The listing builds one solid part. Answer for the finished solid, in the listing's coordinates (mm). Face numbers are marked on the shaded views. A direction names the side the tool comes from. Round coordinates to 2 decimals unless told otherwise and drop trailing zeros. Order: outer loops, then holes, each group sorted by start corner. A loop starts at its lowest first (then second) coordinate and runs counter-clockwise, first axis right, second up. Notation, with made-up numbers: (78.5, -26.75) - (85.5, -26.75) arc R15 ccw to (85.5, -14.75) - close; hole circle Ø10 at (82, 85). An arc over 180 degrees is marked (long way). One line per item, written item: value. Start each with the question number.
1. Section D-D, the plane z = 9.5 is taken. Give the vertices of the cut face in (x, y), then the cut area to 3 significant figures.
2. A tool of negligible diameter and unlimited length cuts with its end or side. For the marked faces 5, 6, 7 and 8, from which of +Z, -Z, +X, -X, +Y, -Y can it reach the whole face along a straight path? Write none if from no direction.
3. Section C-C, the plane y = -0.3 is taken. Give the vertices of the cut face in (x, z).
4. Section B-B, the plane z = -13 is taken. Give the vertices of the cut face in (x, y), then the cut area to 3 significant figures.
5. For a pull along Z with two mould halves and no side action, classify the marked faces 1, 2, 3 and 4 as released by +Z, released by -Z, zero draft, split by the parting line, or undercut.
6. Section A-A, the plane x = 5 is taken. Give the vertices of the cut face in (y, z).
7. Flat-ended cylindrical pins translate along their axes: P1, Ø1.5, axis at y = -0.5, z = 3, coming from the -X side; P2, Ø1.5, axis at x = -7.5, y = 0, coming from the +Z side; P3, Ø1.5, axis at y = -0.5, z = 16, coming from the +X side; P4, Ø4, axis at x = 5, z = 9.5, coming from the +Y side. Find the tip coordinate at first contact, or state that the pin passes through.
8. Straight lines are drawn through the part: line 1 (X direction, y = -0.8, z = 9.5); line 2 (Z direction, x = 1.75, y = -0.95); line 3 (Z direction, x = 5, y = 0.55). For each, find the intervals that lie inside material, in ascending order.
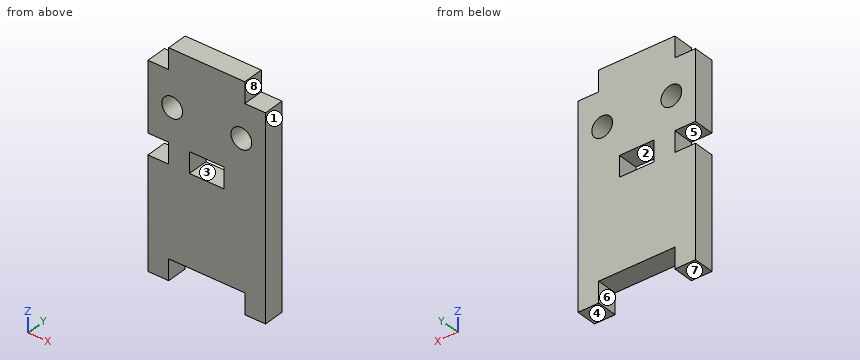
from build123d import *

# Parameters (mm, degrees)
SKETCH1_W               = 17
SKETCH1_H               = 29
BOSS_EXTRUDE1_DEPTH     = 1.5
SKETCH2_W               = 11
SKETCH2_H               = 3
BOSS_EXTRUDE2_DEPTH     = 1.5
SKETCH3_W               = 5
SKETCH3_H               = 3
SKETCH3_W_2             = 11
SKETCH3_W_3             = 3
CUT_EXTRUDE1_DEPTH      = 2.5
CUT_EXTRUDE1_DEPTH_BACK = 2.5
SKETCH5_R               = 1.5
CUT_EXTRUDE3_DEPTH      = 2.5
CUT_EXTRUDE3_DEPTH_BACK = 2.5


with BuildPart() as part:
    # Sketch1 → Boss-Extrude1 (new body, symmetric)
    with BuildSketch(Plane(origin=(0, 0, 0), x_dir=(1, 0, 0), z_dir=(0, 1, 0))):
        Rectangle(SKETCH1_W, SKETCH1_H)
    extrude(amount=BOSS_EXTRUDE1_DEPTH, both=True)

    # Sketch2 → Boss-Extrude2 (add, symmetric)
    with BuildSketch(Plane(origin=(0, 0, 0), x_dir=(1, 0, 0), z_dir=(0, 1, 0))):
        with Locations((0, -16)):
            Rectangle(SKETCH2_W, SKETCH2_H)
    extrude(amount=BOSS_EXTRUDE2_DEPTH, both=True)

    # Sketch3 → Cut-Extrude1 (cut, two sides)
    with BuildSketch(Plane(origin=(0, 0, 0), x_dir=(1, 0, 0), z_dir=(0, 1, 0))) as cut_extrude1_sk:
        with Locations((0, -3)):
            Rectangle(SKETCH3_W, SKETCH3_H)
        with Locations((0, 13)):
            Rectangle(SKETCH3_W_2, SKETCH3_H)
        with Locations((-7, -3)):
            Rectangle(SKETCH3_W_3, SKETCH3_H)
    extrude(amount=CUT_EXTRUDE1_DEPTH, mode=Mode.SUBTRACT)
    extrude(cut_extrude1_sk.sketch, amount=-CUT_EXTRUDE1_DEPTH_BACK, mode=Mode.SUBTRACT)

    # Sketch5 → Cut-Extrude3 (cut, two sides)
    with BuildSketch(Plane(origin=(0, 0, 0), x_dir=(1, 0, 0), z_dir=(0, 1, 0))) as cut_extrude3_sk:
        with Locations((-5, -9.5)):
            Circle(SKETCH5_R)
        with Locations((5, -9.5)):
            Circle(SKETCH5_R)
    extrude(amount=CUT_EXTRUDE3_DEPTH, mode=Mode.SUBTRACT)
    extrude(cut_extrude3_sk.sketch, amount=-CUT_EXTRUDE3_DEPTH_BACK, mode=Mode.SUBTRACT)


solid = part.part
Answer list:
1. outline: (-8.5, -1.5) - (-6.5, -1.5) - (-6.5, 1.5) - (-8.5, 1.5) - close; (-3.5, -1.5) - (3.5, -1.5) - (3.5, 1.5) - (-3.5, 1.5) - close; (6.5, -1.5) - (8.5, -1.5) - (8.5, 1.5) - (6.5, 1.5) - close
1. area: 33.0 mm²
2. face 5: -X, +Y, -Y
2. face 6: -Z, +Y, -Y
2. face 7: -Z, +X, -X, +Y, -Y
2. face 8: +Z, +X, +Y, -Y
3. outline: (-8.5, -14.5) - (-5.5, -14.5) - (-5.5, -11.5) - (5.5, -11.5) - (5.5, -14.5) - (8.5, -14.5) - (8.5, 14.5) - (5.5, 14.5) - (5.5, 17.5) - (-5.5, 17.5) - (-5.5, 14.5) - (-8.5, 14.5) - (-8.5, 4.5) - (-5.5, 4.5) - (-5.5, 1.5) - (-8.5, 1.5) - close; hole circle Ø3 at (-5, 9.5); hole (-2.5, 1.5) - (2.5, 1.5) - (2.5, 4.5) - (-2.5, 4.5) - close; hole circle Ø3 at (5, 9.5)
4. outline: (-8.5, -1.5) - (-5.5, -1.5) - (-5.5, 1.5) - (-8.5, 1.5) - close; (5.5, -1.5) - (8.5, -1.5) - (8.5, 1.5) - (5.5, 1.5) - close
4. area: 18.0 mm²
5. face 1: zero draft
5. face 2: undercut
5. face 3: undercut
5. face 4: released by -Z
6. outline: (-1.5, -11.5) - (1.5, -11.5) - (1.5, 8) - (-1.5, 8) - close; (-1.5, 11) - (1.5, 11) - (1.5, 17.5) - (-1.5, 17.5) - close
7. P1: stops at x = -5.5
7. P2: stops at z = 14.5
7. P3: stops at x = 5.5
7. P4: stops at y = 1.5
8. line 1: x = -8.5 to -6.5, -3.5 to 3.5, 6.5 to 8.5
8. line 2: z = -11.5 to 1.5, 4.5 to 17.5
8. line 3: z = -11.5 to 8, 11 to 17.5
